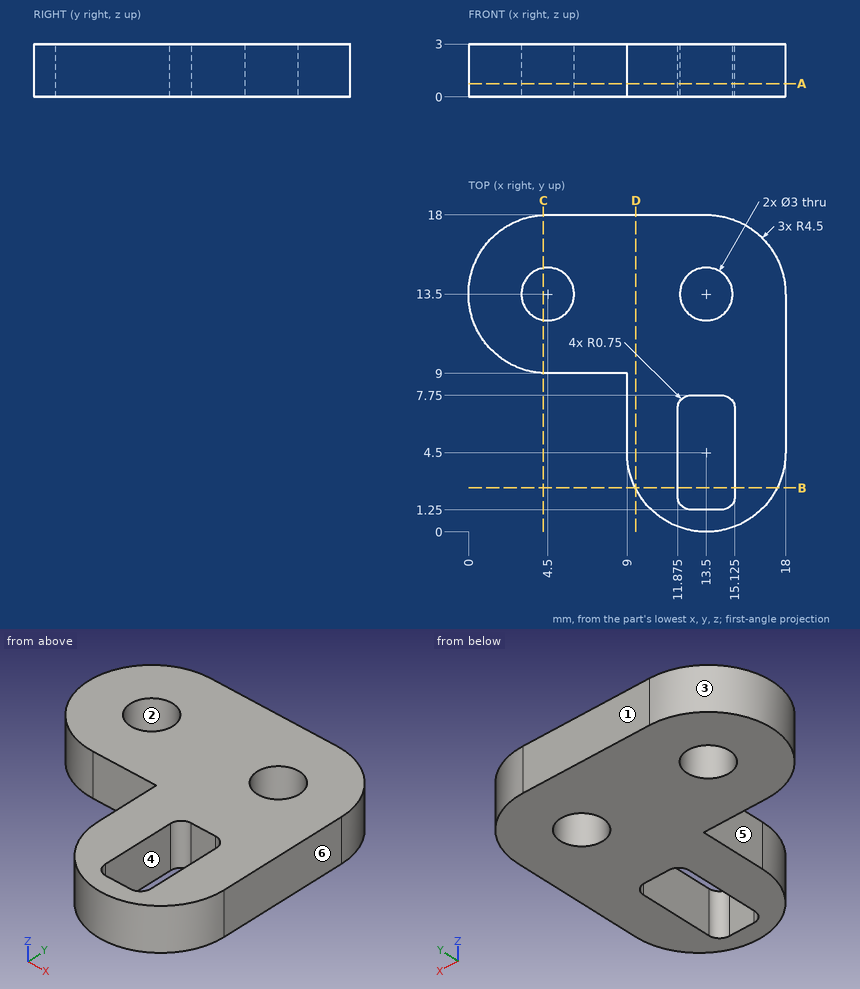
Part print with two shaded views. Sizes in mm from the minimum x, y, z corner. A direction names the side the tool comes from. Give positions to 0.01 mm unless a question says otherwise; leave off trailing zeros. Loops run counter-clockwise (first coordinate to the right, second up) from the corner with the lowest first, then second, coordinate; pieces in that order, holes last. Notation, with made-up numbers: (7, 74) - (25, 74) arc R18 ccw to (25, 100) - close; hole circle Ø4 at (87, 14). An arc over 180 degrees is marked (long way). Put each result on its own line as item: value.
Q1. Flat gauge pins, fed straight in: pin 1 (0.9 mm diameter, centred on x = 7.5, z = 1.5, fed in from -Y); pin 2 (0.5 mm diameter, centred on x = 14, z = 2, fed in from -Y). Where does each tip first touch, or does it go through?
Filled in:
pin 1: stops at y = 9
pin 2: stops at y = 0.01
Q2. Mould opens along Y. For the marked faces 1, 2 and 3 say: pulls with the +Y half, pulls with the -Y half, needs draft (parallel to the pull), parting line crosses it, or undercut.
Filled in:
face 1: pulls with the +Y half
face 2: undercut
face 3: parting line crosses it
Q3. Slice it at D-D (x = 9.5). Give the cut face in (y, z).
Filled in:
outline: (2.44, 0) - (18, 0) - (18, 3) - (2.44, 3) - close
Q4. Slice it at B-B (y = 2.5). Give the cut face in (x, z) (3 decimals).
Filled in:
outline: (9.469, 0) - (11.875, 0) - (11.875, 3) - (9.469, 3) - close; (15.125, 0) - (17.531, 0) - (17.531, 3) - (15.125, 3) - close
Q5. Slice it at C-C (x = 4.25). Give the cut face in (y, z), plus the area to 3 significant figures.
Filled in:
outline: (9.01, 0) - (12.02, 0) - (12.02, 3) - (9.01, 3) - close; (14.98, 0) - (17.99, 0) - (17.99, 3) - (14.98, 3) - close
area: 18.1 mm²
Q6. Slice it at A-A (z = 0.75). Give the cut face in (x, y) (3 decimals).
Filled in:
outline: (4.5, 9) - (9, 9) - (9, 4.5) arc R4.5 ccw to (18, 4.5) - (18, 13.5) arc R4.5 ccw to (13.5, 18) - (4.5, 18) arc R4.5 ccw to start; hole circle Ø3 at (4.5, 13.5); hole (11.875, 2) arc R0.75 ccw to (12.625, 1.25) - (14.375, 1.25) arc R0.75 ccw to (15.125, 2) - (15.125, 7) arc R0.75 ccw to (14.375, 7.75) - (12.625, 7.75) arc R0.75 ccw to (11.875, 7) - close; hole circle Ø3 at (13.5, 13.5)
Q7. Tool access for the marked faces 4, 5 and 6: list every direction of +Z, -Z, +X, -X, +Y, -Y with a clear straight run to the whole face (end or side of a thin tool).
Filled in:
face 4: +Z, -Z
face 5: +Z, -Z, -X, -Y
face 6: +Z, -Z, +X, +Y, -Y
Q8. Probe line 1 along X through (y, z) = (13.5, 1.6); line 2 along Y through (x, z) = (13.5, 1.2); line 3 along Y through (x, z) = (4.5, 0.85). List the from-to ranges inside material, lowest first.
Filled in:
line 1: x = 0 to 3, 6 to 12, 15 to 18
line 2: y = 0 to 1.25, 7.75 to 12, 15 to 18
line 3: y = 9 to 12, 15 to 18
